Work out the finished part from the listing and answer in its coordinate system (mm). A direction names the side the tool comes from. Round coordinates to 2 decimals unless told otherwise and drop trailing zeros. Order: outer loops, then holes, each group sorted by start corner. A loop starts at its lowest first (then second) coordinate and runs counter-clockwise, first axis right, second up. Notation, with made-up numbers: M 73,-29 L 117,-29 A29 cw 117,6 Z; hole C 34,48 d9. An arc over 180 degrees is marked long. Return JSON: item names as keys, results as strings.
from build123d import *

# Parameters (mm, degrees)
F0_W     = 76.2
F0_H     = 127
F0_W_2   = 63.5
F0_H_2   = 114.3
F1_DEPTH = 12.7
F2_W     = 76.2
F2_H     = 127
F3_DEPTH = 6.858
F4_W     = 7.62
F4_H     = 7.62
F5_DEPTH = 63.5
F6_F1_R  = 5.08
F6_F2_R  = 5.08
F6_F3_R  = 5.08
F6_F4_R  = 5.08
F6_F5_R  = 5.08
F6_F6_R  = 5.08
F6_F7_R  = 5.08
F7_R     = 5.08
F8_W     = 12.7
F8_H     = 4.4445483945
F9_DEPTH = 5.588


with BuildPart() as f1:
    # F0 (on Top) → F1 (new body)
    with BuildSketch(Plane.XY):
        Rectangle(F0_W, F0_H)
        Rectangle(F0_W_2, F0_H_2, mode=Mode.SUBTRACT)
    extrude(amount=F1_DEPTH)

    # F2 (on Top) → F3 (join)
    with BuildSketch(Plane.XY):
        Rectangle(F2_W, F2_H)
    extrude(amount=-F3_DEPTH)

    # F4 (on face) → F5 (join)
    with BuildSketch(Plane(origin=(0, 0, -6.858), x_dir=(1, 0, 0), z_dir=(0, 0, -1))):
        with Locations((34.29, -59.69)):
            Rectangle(F4_W, F4_H)
        with Locations((34.29, 59.69)):
            Rectangle(F4_W, F4_H)
        with Locations((-34.29, 59.69)):
            Rectangle(F4_W, F4_H)
        with Locations((-34.29, -59.69)):
            Rectangle(F4_W, F4_H)
    extrude(amount=F5_DEPTH)

    # F6: fillet of radius 5.08 on 7 edges, made by hand

    # F6_f1
    f6_f1_edges = [f1.edges().sort_by_distance(p)[0] for p in [
        (38.1, 55.88, -38.608),
    ]]
    fillet(f6_f1_edges, radius=F6_F1_R)

    # F6_f2
    f6_f2_edges = [f1.edges().sort_by_distance(p)[0] for p in [
        (-38.1, 55.88, -38.608),
    ]]
    fillet(f6_f2_edges, radius=F6_F2_R)

    # F6_f3
    f6_f3_edges = [f1.edges().sort_by_distance(p)[0] for p in [
        (-30.48, -63.5, -38.608),
    ]]
    fillet(f6_f3_edges, radius=F6_F3_R)

    # F6_f4
    f6_f4_edges = [f1.edges().sort_by_distance(p)[0] for p in [
        (38.1, -63.5, -28.829),
    ]]
    fillet(f6_f4_edges, radius=F6_F4_R)

    # F6_f5
    f6_f5_edges = [f1.edges().sort_by_distance(p)[0] for p in [
        (-38.1, -63.5, -28.829),
    ]]
    fillet(f6_f5_edges, radius=F6_F5_R)

    # F6_f6
    f6_f6_edges = [f1.edges().sort_by_distance(p)[0] for p in [
        (38.1, 63.5, -28.829),
    ]]
    fillet(f6_f6_edges, radius=F6_F6_R)

    # F6_f7
    f6_f7_edges = [f1.edges().sort_by_distance(p)[0] for p in [
        (-38.1, 63.5, -28.829),
    ]]
    fillet(f6_f7_edges, radius=F6_F7_R)

    # F7
    f7_edges = [f1.edges().sort_by_distance(p)[0] for p in [
        (-31.75, -57.15, 6.35),
        (31.75, -57.15, 6.35),
        (-31.75, 57.15, 6.35),
        (31.75, 57.15, 6.35),
    ]]
    fillet(f7_edges, radius=F7_R)

    # F8 (on face) → F9 (cut)
    with BuildSketch(Plane.XZ.offset(-57.15)):
        with Locations((-6.35, 2.2222741973)):
            Rectangle(F8_W, F8_H)
    extrude(amount=-F9_DEPTH, mode=Mode.SUBTRACT)


solid = f1.part
Item 1: Each of these flat-tipped pins is pushed along its axis until it touches: pin 1 (3 mm diameter, centred on x = -1.5, y = -16, fed in from +Z); pin 2 (2 mm diameter, centred on y = 61, z = 3, fed in from +X); pin 3 (2 mm diameter, centred on x = -31.5, z = -38, fed in from -Y) (3 decimals). Where does it stop, or does it pass through?
Output:
{"pin 1": "stops at z = 0", "pin 2": "stops at x = 37.85", "pin 3": "stops at y = -62.475"}
Item 2: Find section D-D (x = -4.5). Determine the outline of the cut face in (y, z), plus the area to 3 significant figures.
Output:
{"outline": "M -63.5,-6.86 L 63.5,-6.86 L 63.5,12.7 L 57.15,12.7 L 57.15,4.44 L 62.74,4.44 L 62.74,0 L -57.15,0 L -57.15,12.7 L -63.5,12.7 Z", "area": "1,010 mm^2"}
Item 3: Find section C-C (y = -5). Determine the outline of the cut face in (x, z).
Output:
{"outline": "M -38.1,-6.86 L 38.1,-6.86 L 38.1,12.7 L 31.75,12.7 L 31.75,0 L -31.75,0 L -31.75,12.7 L -38.1,12.7 Z"}
Item 4: The mould has two halves that part along X. Classify faces 1 (the flat face through (0, -57.15, 6)), 2 (the flat face through (33, 60, -70.358)), 3 (the cylindrical face through (-36.572, 62.051, -28.248)): pulls with the +X half, pulls with the -X half, needs draft (parallel to the pull), parting line crosses it, or undercut.
Output:
{"face 1": "undercut", "face 2": "needs draft", "face 3": "pulls with the -X half"}
Item 5: Find section A-A (z = -54.5). Determine the outline of the cut face in (x, y).
Output:
{"outline": "M -38.1,-58.42 A5.08 ccw -34.29,-63.34 A5.08 ccw -30.48,-58.42 L -30.48,-55.88 L -38.1,-55.88 Z; M -37.94,59.69 A5.08 ccw -33.02,55.88 L -30.48,55.88 L -30.48,63.5 L -33.02,63.5 A5.08 ccw Z; M 30.48,-63.5 L 33.02,-63.5 A5.08 ccw 38.1,-58.42 L 38.1,-55.88 L 30.48,-55.88 Z; M 30.48,55.88 L 33.02,55.88 A5.08 ccw 37.94,59.69 A5.08 ccw 33.02,63.5 L 30.48,63.5 Z"}
Item 6: Which of the six approach directions +Z, -Z, +X, -X, +Y, -Y give full straight-line access (tool end or side, diameter ignored) to faces 4 (the cylindrical face through (-36.2, 57, -39.1)), 5 (the flat face through (34, -55.88, -38)), 6 (the cylindrical face through (30.301, 55.622, 6.439))?
Output:
{"face 4": "-Z, -X", "face 5": "-Z, +X, -X", "face 6": "+Z"}
Item 7: Find section B-B (x = 18.5). Determine the outline of the cut face in (y, z), plus the area to 3 significant figures.
Output:
{"outline": "M -63.5,-6.86 L 63.5,-6.86 L 63.5,12.7 L 57.15,12.7 L 57.15,0 L -57.15,0 L -57.15,12.7 L -63.5,12.7 Z", "area": "1,030 mm^2"}
Item 8: Consider line 1 along Y through (x, z) = (0.5, 3); line 2 along Y through (x, z) = (32.5, -16); line 3 along X through (y, z) = (-57.5, -58.5). Determine where each line is inside the solid, lowest interval first. Write a range as [from, to].
Output:
{"line 1": "y = [-63.5, -57.15], [57.15, 63.5]", "line 2": "y = [-63.5, -55.88], [55.88, 63.5]", "line 3": "x = [-38.1, -30.48], [30.48, 38.1]"}
